```python
from build123d import *

# Parameters (mm, degrees)
BOSS_EXTRUDE1_DEPTH = 3


with BuildPart() as part:
    # Sketch1 → Boss-Extrude1 (new body)
    with BuildSketch(Plane(origin=(0, 0, 0), x_dir=(1, 0, 0), z_dir=(0, 1, 0))):
        with BuildLine():
            ThreePointArc((2.75, 0), (2.542144764, 1.048808848), (1.95, 1.939071943))
            Line((1.95, 1.939071943), (1.95, -1.939071943))
            ThreePointArc((1.95, -1.939071943), (2.542144764, -1.048808848), (2.75, 0))
        make_face()
        with BuildLine():
            ThreePointArc((1.95, 5.674284096), (0, 6), (-1.95, 5.674284096))
            Line((-1.95, 5.674284096), (-1.95, 1.939071943))
            ThreePointArc((-1.95, 1.939071943), (0, 2.75), (1.95, 1.939071943))
            Line((1.95, 1.939071943), (1.95, 5.674284096))
        make_face()
        with BuildLine():
            Line((-1.95, -1.939071943), (-1.95, -5.674284096))
            ThreePointArc((-1.95, -5.674284096), (0, -6), (1.95, -5.674284096))
            Line((1.95, -5.674284096), (1.95, -1.939071943))
            ThreePointArc((1.95, -1.939071943), (0, -2.75), (-1.95, -1.939071943))
        make_face()
        with BuildLine():
            Line((-1.95, 1.939071943), (-1.95, 5.674284096))
            ThreePointArc((-1.95, 5.674284096), (-6, 0), (-1.95, -5.674284096))
            Line((-1.95, -5.674284096), (-1.95, -1.939071943))
            ThreePointArc((-1.95, -1.939071943), (-2.75, 0), (-1.95, 1.939071943))
        make_face()
        with BuildLine():
            ThreePointArc((6, 0), (4.883646179, 3.485685012), (1.95, 5.674284096))
            Line((1.95, 5.674284096), (1.95, 1.939071943))
            ThreePointArc((1.95, 1.939071943), (2.542144764, 1.048808848), (2.75, 0))
            ThreePointArc((2.75, 0), (2.542144764, -1.048808848), (1.95, -1.939071943))
            Line((1.95, -1.939071943), (1.95, -5.674284096))
            ThreePointArc((1.95, -5.674284096), (4.883646179, -3.485685012), (6, 0))
        make_face()
        with BuildLine():
            Line((-1.95, -1.939071943), (-1.95, 1.939071943))
            ThreePointArc((-1.95, 1.939071943), (-2.75, 0), (-1.95, -1.939071943))
        make_face()
    extrude(amount=BOSS_EXTRUDE1_DEPTH)


solid = part.part
```
The model under review builds one solid part; all positions refer to its coordinate system, in mm. A direction names the side the tool comes from. Round coordinates to 2 decimals unless told otherwise and drop trailing zeros. Order: outer loops, then holes, each group sorted by start corner. A loop starts at its lowest first (then second) coordinate and runs counter-clockwise, first axis right, second up. Notation, with made-up numbers: (-18, 74.25) - (10, 74.25) arc R18 ccw to (10, 96.25) - close; hole circle Ø8 at (8.25, 36). An arc over 180 degrees is marked (long way). Answer in a Markdown table with one row per item.
(1) Take a section at B-B on z = 1.5. Write out the cut boundary in (x, y).
Result set:
| item | result |
|---|---|
| outline | (-5.81, 0) - (-1.95, 0) - (-1.95, 3) - (-5.81, 3) - close; (1.95, 0) - (5.81, 0) - (5.81, 3) - (1.95, 3) - close |
(2) Machinability: for faces 3 (the face through (-1.95, 1, 0)), 4 (the face through (3, 3, 0)), which of the approach directions +Z, -Z, +X, -X, +Y, -Y give a long, thin tool a straight path to every point of the face, cutting with its end or side? Answer none if there is none.
Result set:
| item | result |
|---|---|
| face 3 | +Y, -Y |
| face 4 | +Z, -Z, +X, -X, +Y |
(3) Take a section at A-A on y = 1.9. Write out the cut boundary in (x, z), plus the area to 3 significant figures.
Result set:
| item | result |
|---|---|
| outline | circle Ø12 at (0, 0); hole (-1.95, -1.94) arc R2.75 ccw to (1.95, -1.94) - (1.95, 1.94) arc R2.75 ccw to (-1.95, 1.94) - close |
| area | 93.6 mm2 |
(4) For line 1 (X direction, y = 0.65, z = -0.5); line 2 (X direction, y = 2.05, z = -1.5); line 3 (Z direction, x = 1, y = 1.35), list the stretches that pass through material, from the lowest coordinate up. Write a range as from..to.
Result set:
| item | result |
|---|---|
| line 1 | x = -5.98..-1.95, 1.95..5.98 |
| line 2 | x = -5.81..-1.95, 1.95..5.81 |
| line 3 | z = -5.92..-2.56, 2.56..5.92 |
(5) Clearance check with a flat-ended pin moving along its axis: P1, Ø1, axis at y = 1, z = -2, coming from the +X side. State where the tip first meets the part, or that it passes through.
Result set:
| item | result |
|---|---|
| P1 | stops at x = 5.81 |
(6) Mouldability with a two-part tool opening along Z and no side actions: class faces 1 (the face through (3, 0, 0)), 2 (the face through (0.03, 1.48, 2.75)) as released by +Z, released by -Z, zero draft, split by the parting line, or undercut.
Result set:
| item | result |
|---|---|
| face 1 | zero draft |
| face 2 | undercut |
(7) Take a section at D-D on x = 2.25. Write out the cut boundary in (y, z).
Result set:
| item | result |
|---|---|
| outline | (0, -5.56) - (3, -5.56) - (3, 5.56) - (0, 5.56) - close |
(8) Take a section at C-C on x = 1. Write out the cut boundary in (y, z).
Result set:
| item | result |
|---|---|
| outline | (0, -5.92) - (3, -5.92) - (3, -2.56) - (0, -2.56) - close; (0, 2.56) - (3, 2.56) - (3, 5.92) - (0, 5.92) - close |
